The model under review builds one solid part; all positions refer to its coordinate system, in mm. Face numbers are marked on the shaded views. A direction names the side the tool comes from. Round coordinates to 2 decimals unless told otherwise and drop trailing zeros. Return JSON: item names as keys, results as strings.
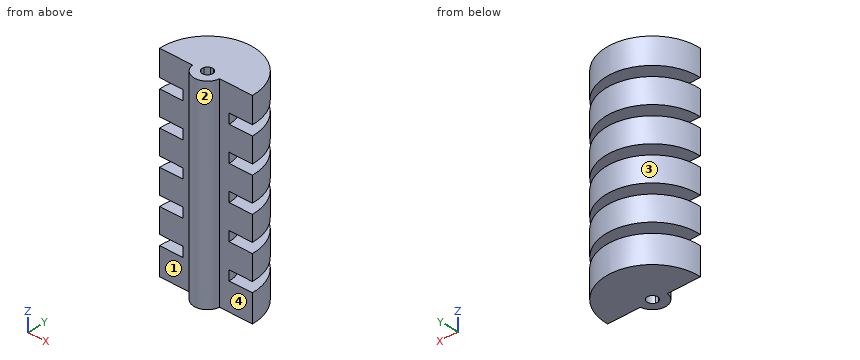
from build123d import *

# Parameters (mm, degrees)
SKETCH3_R            = 27.94
BOSS_EXTRUDE2_DEPTH  = 122.46
SKETCH5_R            = 3.175
CUT_EXTRUDE1_DEPTH   = 129.676877488
SKETCH4_W            = 14
SKETCH4_H            = 6
SHELL1_START         = 3
SHELL1_OUTLINE_R     = 10.94
SHELL1_OUTLINE_R_2   = 6.175
SHELL1_DEPTH         = 116.46
SHELL1_2_OUTLINE_R   = 24.94
SHELL1_2_OUTLINE_R_2 = 10.94
SHELL1_2_DEPTH       = 10.72
SHELL1_START_2       = 109.72
SHELL1_3_OUTLINE_R   = 24.94
SHELL1_3_OUTLINE_R_2 = 10.94
SHELL1_3_DEPTH       = 9.74
SHELL1_START_3       = 25.72
SHELL1_4_OUTLINE_R   = 24.94
SHELL1_4_OUTLINE_R_2 = 10.94
SHELL1_4_DEPTH       = 9
SHELL1_START_4       = 46.72
SHELL1_5_OUTLINE_R   = 24.94
SHELL1_5_OUTLINE_R_2 = 10.94
SHELL1_5_DEPTH       = 9
SHELL1_START_5       = 67.72
SHELL1_6_OUTLINE_R   = 24.94
SHELL1_6_OUTLINE_R_2 = 10.94
SHELL1_6_DEPTH       = 9
SHELL1_START_6       = 88.72
SHELL1_7_OUTLINE_R   = 24.94
SHELL1_7_OUTLINE_R_2 = 10.94
SHELL1_7_DEPTH       = 9
BOSS_EXTRUDE3_REACH  = 130.677
SKETCH13_W           = 16.483162312
SKETCH13_H           = 6
CUT_EXTRUDE3_DEPTH   = 123
BOSS_EXTRUDE5_START  = -122.46
BOSS_EXTRUDE5_DEPTH  = 122.46


# Read off the part's stored shape, not the designer's step: Shell1
with BuildPart() as part:
    # Sketch3 → Boss-Extrude2 (new body)
    with BuildSketch(Plane.XY):
        Circle(SKETCH3_R)
    extrude(amount=BOSS_EXTRUDE2_DEPTH)

    # Sketch5 → Cut-Extrude1 (cut, through all)
    with BuildSketch(Plane.XY.offset(122.46)):
        Circle(SKETCH5_R)
    extrude(amount=-CUT_EXTRUDE1_DEPTH, mode=Mode.SUBTRACT)

    # Sketch4 → Cut-Revolve1 (revolve, cut)
    with BuildSketch(Plane(origin=(0, 0, 0), x_dir=(1, 0, 0), z_dir=(0, 1, 0)), mode=Mode.PRIVATE) as cut_revolve1_sk:
        with Locations((-20.94, -103.72)):
            Rectangle(SKETCH4_W, SKETCH4_H)
        with Locations((-20.94, -82.72)):
            Rectangle(SKETCH4_W, SKETCH4_H)
        with Locations((-20.94, -61.72)):
            Rectangle(SKETCH4_W, SKETCH4_H)
        with Locations((-20.94, -40.72)):
            Rectangle(SKETCH4_W, SKETCH4_H)
        with Locations((-20.94, -19.72)):
            Rectangle(SKETCH4_W, SKETCH4_H)
    revolve(cut_revolve1_sk.sketch.rotate(Axis((0, 0, 122.46), (0, 0, -1)), 180), axis=Axis((0, 0, 122.46), (0, 0, -1)), mode=Mode.SUBTRACT)

    # Shell1 outline → Shell1 (cut)
    with BuildSketch(Plane.XY.offset(SHELL1_START)):
        Circle(SHELL1_OUTLINE_R)
        Circle(SHELL1_OUTLINE_R_2, mode=Mode.SUBTRACT)
    extrude(amount=SHELL1_DEPTH, mode=Mode.SUBTRACT)

    # Shell1 2 outline → Shell1 2 (cut)
    with BuildSketch(Plane.XY.offset(SHELL1_START)):
        Circle(SHELL1_2_OUTLINE_R)
        Circle(SHELL1_2_OUTLINE_R_2, mode=Mode.SUBTRACT)
    extrude(amount=SHELL1_2_DEPTH, mode=Mode.SUBTRACT)

    # Shell1 3 outline → Shell1 3 (cut)
    with BuildSketch(Plane.XY.offset(SHELL1_START_2)):
        Circle(SHELL1_3_OUTLINE_R)
        Circle(SHELL1_3_OUTLINE_R_2, mode=Mode.SUBTRACT)
    extrude(amount=SHELL1_3_DEPTH, mode=Mode.SUBTRACT)

    # Shell1 4 outline → Shell1 4 (cut)
    with BuildSketch(Plane.XY.offset(SHELL1_START_3)):
        Circle(SHELL1_4_OUTLINE_R)
        Circle(SHELL1_4_OUTLINE_R_2, mode=Mode.SUBTRACT)
    extrude(amount=SHELL1_4_DEPTH, mode=Mode.SUBTRACT)

    # Shell1 5 outline → Shell1 5 (cut)
    with BuildSketch(Plane.XY.offset(SHELL1_START_4)):
        Circle(SHELL1_5_OUTLINE_R)
        Circle(SHELL1_5_OUTLINE_R_2, mode=Mode.SUBTRACT)
    extrude(amount=SHELL1_5_DEPTH, mode=Mode.SUBTRACT)

    # Shell1 6 outline → Shell1 6 (cut)
    with BuildSketch(Plane.XY.offset(SHELL1_START_5)):
        Circle(SHELL1_6_OUTLINE_R)
        Circle(SHELL1_6_OUTLINE_R_2, mode=Mode.SUBTRACT)
    extrude(amount=SHELL1_6_DEPTH, mode=Mode.SUBTRACT)

    # Shell1 7 outline → Shell1 7 (cut)
    with BuildSketch(Plane.XY.offset(SHELL1_START_6)):
        Circle(SHELL1_7_OUTLINE_R)
        Circle(SHELL1_7_OUTLINE_R_2, mode=Mode.SUBTRACT)
    extrude(amount=SHELL1_7_DEPTH, mode=Mode.SUBTRACT)

    # Boss-Extrude3: up to this face of the body (flat: up to its plane)
    boss_extrude3_end = Plane(part.part.faces().sort_by_distance((-27.149737461, 0, 122.46))[0])
    # Sketch10 → Boss-Extrude3 (add, up to the picked face)
    with BuildSketch(Plane(origin=(0, 0, 0), x_dir=(-1, 0, 0), z_dir=(0, 0, -1)), mode=Mode.PRIVATE) as boss_extrude3_sk1:
        with BuildLine():
            Line((-1, 27.922098775), (-1, 3.01340754))
            ThreePointArc((-1, 3.01340754), (0, 3.175), (1, 3.01340754))
            Line((1, 3.01340754), (1, 27.922098775))
            ThreePointArc((1, 27.922098775), (0, 27.94), (-1, 27.922098775))
        make_face()
    boss_extrude3_tool1 = split(extrude(boss_extrude3_sk1.sketch, amount=-BOSS_EXTRUDE3_REACH, mode=Mode.PRIVATE), bisect_by=boss_extrude3_end, keep=Keep.BOTH, mode=Mode.PRIVATE)
    # Sketch10 → Boss-Extrude3 (add, up to the picked face)
    with BuildSketch(Plane(origin=(0, 0, 0), x_dir=(-1, 0, 0), z_dir=(0, 0, -1)), mode=Mode.PRIVATE) as boss_extrude3_sk2:
        with BuildLine():
            Line((3.01340754, 1), (27.922098775, 1))
            ThreePointArc((27.922098775, 1), (27.94, 0), (27.922098775, -1))
            Line((27.922098775, -1), (3.01340754, -1))
            ThreePointArc((3.01340754, -1), (3.175, 0), (3.01340754, 1))
        make_face()
    boss_extrude3_tool2 = split(extrude(boss_extrude3_sk2.sketch, amount=-BOSS_EXTRUDE3_REACH, mode=Mode.PRIVATE), bisect_by=boss_extrude3_end, keep=Keep.BOTH, mode=Mode.PRIVATE)
    # Sketch10 → Boss-Extrude3 (add, up to the picked face)
    with BuildSketch(Plane(origin=(0, 0, 0), x_dir=(-1, 0, 0), z_dir=(0, 0, -1)), mode=Mode.PRIVATE) as boss_extrude3_sk3:
        with BuildLine():
            Line((-1, -3.01340754), (-1, -27.922098775))
            ThreePointArc((-1, -27.922098775), (0, -27.94), (1, -27.922098775))
            Line((1, -27.922098775), (1, -3.01340754))
            ThreePointArc((1, -3.01340754), (0, -3.175), (-1, -3.01340754))
        make_face()
    boss_extrude3_tool3 = split(extrude(boss_extrude3_sk3.sketch, amount=-BOSS_EXTRUDE3_REACH, mode=Mode.PRIVATE), bisect_by=boss_extrude3_end, keep=Keep.BOTH, mode=Mode.PRIVATE)
    # Sketch10 → Boss-Extrude3 (add, up to the picked face)
    with BuildSketch(Plane(origin=(0, 0, 0), x_dir=(-1, 0, 0), z_dir=(0, 0, -1)), mode=Mode.PRIVATE) as boss_extrude3_sk4:
        with BuildLine():
            Line((-27.922098775, -1), (-3.01340754, -1))
            ThreePointArc((-3.01340754, -1), (-3.175, 0), (-3.01340754, 1))
            Line((-3.01340754, 1), (-27.922098775, 1))
            ThreePointArc((-27.922098775, 1), (-27.94, 0), (-27.922098775, -1))
        make_face()
    boss_extrude3_tool4 = split(extrude(boss_extrude3_sk4.sketch, amount=-BOSS_EXTRUDE3_REACH, mode=Mode.PRIVATE), bisect_by=boss_extrude3_end, keep=Keep.BOTH, mode=Mode.PRIVATE)
    add(boss_extrude3_tool1.solids().sort_by(Axis((0, 15.527819, 0), (0, 0, 1)))[0])
    add(boss_extrude3_tool2.solids().sort_by(Axis((-15.527819, 0, 0), (0, 0, 1)))[0])
    add(boss_extrude3_tool3.solids().sort_by(Axis((0, -15.527819, 0), (0, 0, 1)))[0])
    add(boss_extrude3_tool4.solids().sort_by(Axis((15.527819, 0, 0), (0, 0, 1)))[0])

    # Sketch13 → Cut-Revolve2 (revolve, cut)
    with BuildSketch(Plane(origin=(0, 0, 0), x_dir=(1, 0, 0), z_dir=(0, 1, 0)), mode=Mode.PRIVATE) as cut_revolve2_sk:
        with Locations((-22.145666886, -40.72)):
            Rectangle(SKETCH13_W, SKETCH13_H)
        with Locations((-22.145666886, -19.72)):
            Rectangle(SKETCH13_W, SKETCH13_H)
        with Locations((-22.145666886, -61.72)):
            Rectangle(SKETCH13_W, SKETCH13_H)
        with Locations((-22.145666886, -82.72)):
            Rectangle(SKETCH13_W, SKETCH13_H)
        with Locations((-22.145666886, -103.72)):
            Rectangle(SKETCH13_W, SKETCH13_H)
    revolve(cut_revolve2_sk.sketch.rotate(Axis((0, 0, 121.588746248), (0, 0, -1)), 180), axis=Axis((0, 0, 121.588746248), (0, 0, -1)), mode=Mode.SUBTRACT)

    # Sketch16 → Cut-Extrude3 (cut)
    with BuildSketch(Plane(origin=(0, 0, 0), x_dir=(-1, 0, 0), z_dir=(0, 0, -1))):
        with BuildLine():
            Line((-27.923120749, -0.971044624), (-6.098171639, -0.971044624))
            ThreePointArc((-6.098171639, -0.971044624), (-0.014665674, -6.174982584), (6.093490379, -1))
            Line((6.093490379, -1), (27.922098775, -1))
            ThreePointArc((27.922098775, -1), (-0.014486703, -27.939996244), (-27.923120749, -0.971044624))
        make_face()
    extrude(amount=-CUT_EXTRUDE3_DEPTH, mode=Mode.SUBTRACT)

    # Sketch18 → Boss-Extrude5 (add)
    with BuildSketch(Plane(origin=(0, 0, 0), x_dir=(-1, 0, 0), z_dir=(0, 0, -1)).offset(BOSS_EXTRUDE5_START)):
        with BuildLine():
            Line((-3.175, 0), (-8.175, 0))
            ThreePointArc((-8.175, 0), (0, -8.175), (8.175, 0))
            Line((8.175, 0), (3.175, 0))
            ThreePointArc((3.175, 0), (0, -3.175), (-3.175, 0))
        make_face()
    extrude(amount=BOSS_EXTRUDE5_DEPTH)


solid = part.part
(1) Wall thickness on line 1 (X direction, y = 2, z = 73.5); line 2 (X direction, y = 12.5, z = 70); line 3 (X direction, y = 9, z = 114): over which ranges is each line inside the solid? List them lowest first.
Filled in:
{"line 1": "x = -27.87 to -24.86, -5.84 to -2.47, 2.47 to 5.84, 24.86 to 27.87", "line 2": "x = -24.99 to -21.58, -1 to 1, 21.58 to 24.99", "line 3": "x = -26.45 to -23.26, -1 to 1, 23.26 to 26.45"}
(2) For the marked faces 1 and 2, list the 3-axis set-ups (+Z, -Z, +X, -X, +Y, -Y) from which the entire face can be reached by the end or side of a thin tool; tool diameter is ignored.
Filled in:
{"face 1": "+Z, -Z, -X, -Y", "face 2": "+Z, -Z, -Y"}
(3) Add section A-A (z = 81). Give the number of separate pieces and of enclosed holes in the cut face, plus the area to 3 significant figures.
Filled in:
{"separate pieces": "1", "enclosed holes": "3", "area": "279 mm2"}
(4) Clearance check with flat-ended pins moving along their axes: pin 1 Ø7 at (x, y) = (-14.5, 7.5) entering from -Z; pin 2 Ø10 at (x, z) = (-9, 105) entering from -Y; pin 3 Ø3 at (x, z) = (-18.5, 57.5) entering from +Y; pin 4 Ø4 at (y, z) = (14.5, 44.5) entering from +X. State where each tip first meets the part, or that it passes through.
Filled in:
{"pin 1": "stops at z = 0", "pin 2": "stops at y = -7.13", "pin 3": "stops at y = 22.17", "pin 4": "stops at x = 24.99"}
(5) Mouldability with a two-part tool opening along X and no side actions: class the marked faces 3 and 4 as released by +X, released by -X, zero draft, split by the parting line, or undercut.
Filled in:
{"face 3": "split by the parting line", "face 4": "zero draft"}
